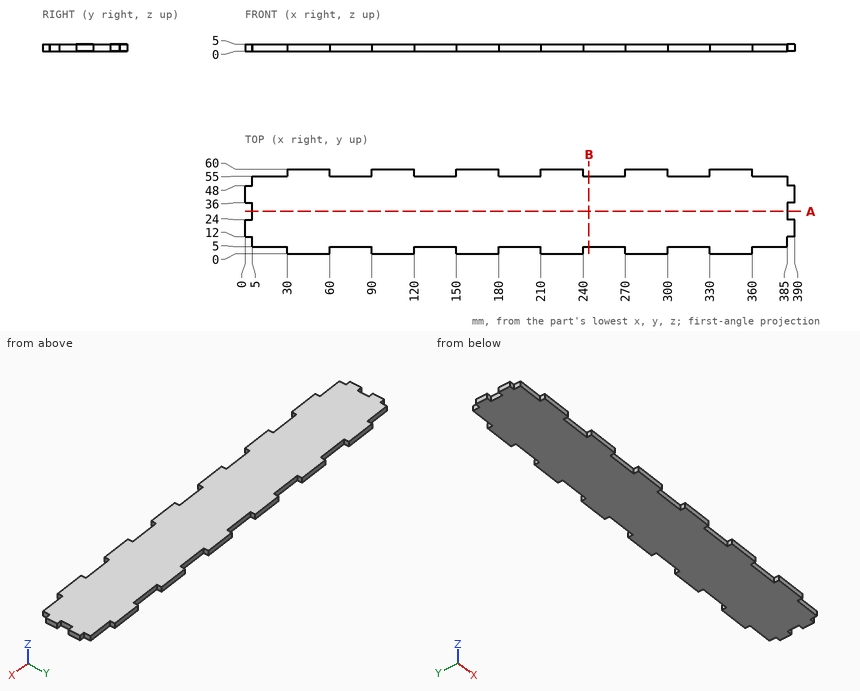
Drawing for the job (mm, zero at the part's lowest x, y, z). Round coordinates to 2 decimals unless told otherwise and drop trailing zeros. Loops run counter-clockwise (first coordinate to the right, second up) from the corner with the lowest first, then second, coordinate; pieces in that order, holes last. Notation, with made-up numbers: (-11.75, 6.5) -> (29.25, 6.5) arc R19 cw to (29.25, 33.5) -> close; hole circle Ø11 at (4, 44). An arc over 180 degrees is marked (long way). Use one line per item in the form item = value. Start each with the question number.
Item 1: Band-saw the part on B-B (x = 244). List the corners of the cut face in (y, z), plus the area to 3 significant figures.
Item 2: Band-saw the part on A-A (y = 30). List the corners of the cut face in (x, z), plus the area to 3 significant figures.
Item 3: Drop flat-ended pins along their axis: pin 1 Ø1.5 at (x, z) = (387.5, 1.5) entering from -Y; pin 2 Ø2.5 at (x, z) = (310.5, 1.5) entering from +Y; pin 3 Ø1.5 at (y, z) = (58, 2) entering from +X; pin 4 Ø2 at (y, z) = (19, 2.5) entering from -X. Give the stop position or say it passes through.
Item 4: Drill centre lines: line 1 along X through (y, z) = (3, 1.7); line 2 along X through (y, z) = (10.5, 2.7); line 3 along Y through (x, z) = (367, 1.5). Where is each one in solid material? Low to high.
Data:
q1.outline = (5, 0) -> (55, 0) -> (55, 5) -> (5, 5) -> close
q1.area = 250 mm^2
q2.outline = (5, 0) -> (385, 0) -> (385, 5) -> (5, 5) -> close
q2.area = 1,900 mm^2
q3.pin_1 = 12
q3.pin_2 = 55
q3.pin_3 = 360
q3.pin_4 = 0
q4.line_1 = 30 to 60, 90 to 120, 150 to 180, 210 to 240, 270 to 300, 330 to 360
q4.line_2 = 5 to 385
q4.line_3 = 5 to 55
